Verification items for this drawing (mm, ordinates from the low corner). Give positions to 0.01 mm unless a question says otherwise; leave off trailing zeros. Loops run counter-clockwise (first coordinate to the right, second up) from the corner with the lowest first, then second, coordinate; pieces in that order, holes last. Notation, with made-up numbers: (84.25, 14.25) - (103.25, 14.25) arc R16 cw to (103.25, 19.25) - close; hole circle Ø9 at (-21, 23). An arc over 180 degrees is marked (long way). Write item = value, one per line. Start each with the question number.
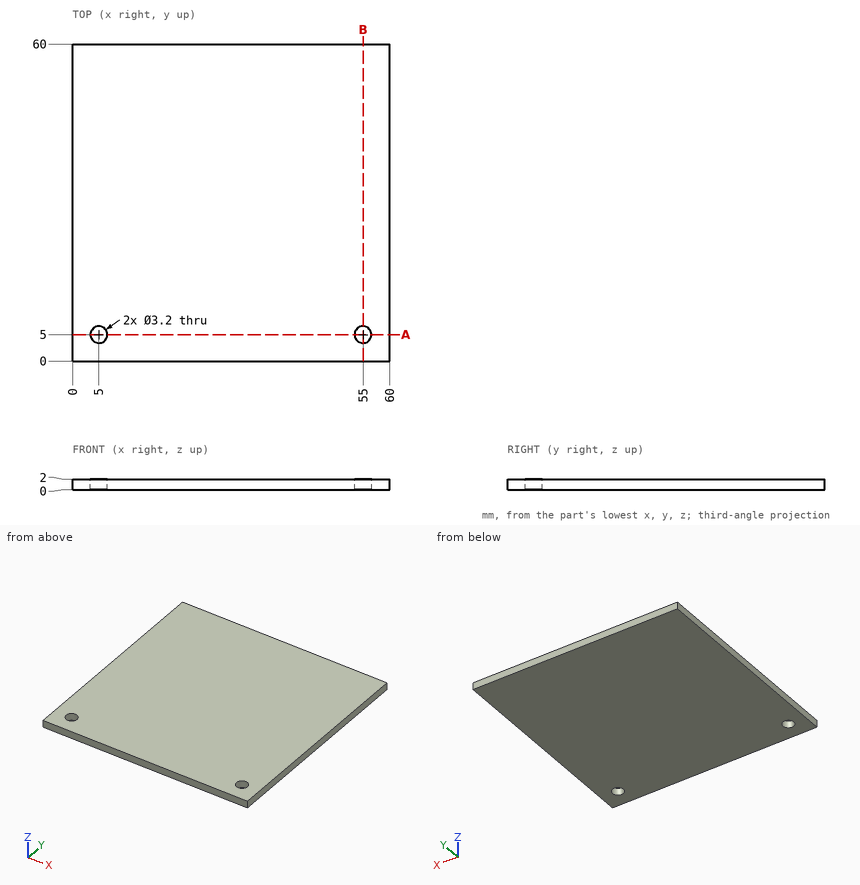
1) Cross-section at A-A on y = 5. Enter the section's corners in (x, z), and give its area (3 significant figures).
2) Material ranges on line 1 along Y through (x, z) = (5, 1.6), recorded low to high.
3) Cross-section at B-B on x = 55. Enter the section's corners in (y, z), and give its area (3 significant figures).
4) Gauge pin test, flat end, axial feed: P1, Ø8, axis at x = 46, y = 12, coming from the -Z side. Record the tip position at first contact, or that the pin passes through.
Checked values:
q1.outline = (0, 0) - (3.4, 0) - (3.4, 2) - (0, 2) - close; (6.6, 0) - (53.4, 0) - (53.4, 2) - (6.6, 2) - close; (56.6, 0) - (60, 0) - (60, 2) - (56.6, 2) - close
q1.area = 107 mm²
q2.line_1 = 0 to 3.4, 6.6 to 60
q3.outline = (0, 0) - (3.4, 0) - (3.4, 2) - (0, 2) - close; (6.6, 0) - (60, 0) - (60, 2) - (6.6, 2) - close
q3.area = 114 mm²
q4.P1 = 0
